```python
from build123d import *

# Parameters (mm, degrees)
F0_W      = 160
F0_H      = 35
F1_DEPTH  = 5
F3_D      = 4.5
F5_R      = 9
F6_DEPTH  = 20
F8_DEPTH  = 25
F9_W      = 15
F9_H      = 2
F10_DEPTH = 20
F12_D     = 4.5
F12_DEPTH = 12
F12_TIP   = 1.3519363928


with BuildPart() as f1:
    # F0 (on Top) → F1 (new body)
    with BuildSketch(Plane.XY):
        with Locations((80, 17.5)):
            Rectangle(F0_W, F0_H)
    extrude(amount=F1_DEPTH)

    # F3 (through all)
    with Locations(Plane(origin=(0, 0, 0), x_dir=(1, 0, 0), z_dir=(0, 0, -1))):
        with Locations((20, -9.5), (60, -9.5), (60, -25.5), (20, -25.5)):
            Hole(F3_D / 2)

    # F5 (on offset) → F6 (join)
    with BuildSketch(Plane.YZ.offset(120)):
        with BuildLine():
            Line((5, 23), (5, 5))
            Line((5, 5), (30, 5))
            Line((30, 5), (30, 23))
            ThreePointArc((30, 23), (17.5, 35.5), (5, 23))
        make_face()
        with Locations((17.5, 23)):
            Circle(F5_R, mode=Mode.SUBTRACT)
    extrude(amount=F6_DEPTH)

    # F7 (on face) → F8 (cut)
    with BuildSketch(Plane.YZ.offset(140)):
        with BuildLine():
            Line((29.9599357944, 24), (26.44427191, 24))
            ThreePointArc((26.44427191, 24), (26.4860571774, 23.5007758031), (26.5, 23))
            ThreePointArc((26.5, 23), (26.4860571774, 22.4992241969), (26.44427191, 22))
            Line((26.44427191, 22), (30, 22))
            Line((30, 22), (30, 23))
            ThreePointArc((30, 23), (29.9899799325, 23.5004011242), (29.9599357944, 24))
        make_face()
    extrude(amount=-F8_DEPTH, mode=Mode.SUBTRACT)

    # F9 (on offset) → F10 (join)
    with BuildSketch(Plane.YZ.offset(120)):
        with Locations((36, 21)):
            Rectangle(F9_W, F9_H)
        with Locations((36, 25)):
            Rectangle(F9_W, F9_H)
    extrude(amount=F10_DEPTH)

    # F12
    with Locations(Plane.XY.offset(26)):
        with Locations((130, 36)):
            Hole(F12_D / 2, depth=F12_DEPTH)
            with Locations((0, 0, -(F12_DEPTH + F12_TIP / 2))):  # 118° drill point
                Cone(0, F12_D / 2, F12_TIP, mode=Mode.SUBTRACT)


solid = f1.part
```
Can you work these out from the model? Positions are in its coordinate system, mm. A direction names the side the tool comes from. Round coordinates to 2 decimals unless told otherwise and drop trailing zeros. Loops run counter-clockwise (first coordinate to the right, second up) from the corner with the lowest first, then second, coordinate; pieces in that order, holes last. Notation, with made-up numbers: (60, 34.5) -> (97, 34.5) arc R20 cw to (97, 64.5) -> close; hole circle Ø1 at (31.5, 10.25). An arc over 180 degrees is marked (long way). Answer in a Markdown table with one row per item.
Item 1: Will these pins go through, and if not, where does the flat tip stop? P1, Ø14.5, axis at x = 132.5, z = 13.5, coming from the -Y side; P2, Ø4, axis at x = 60, y = 25.5, coming from the +Z side; P3, Ø3, axis at x = 135, y = 9, coming from the +Z side; P4, Ø4, axis at x = 126.5, y = 35.5, coming from the +Z side.
Answer block:
| item | result |
|---|---|
| P1 | y = 5 |
| P2 | through |
| P3 | z = 33.36 |
| P4 | z = 26 |
Item 2: On a 3-axis mill with a long thin cutter (end or side, diameter ignored), from which of +Z, -Z, +X, -X, +Y, -Y can I reach the whole of each face in a straight line? I mean faces 5 (the flat face through (127.6, 36.7, 20)), 6 (the flat face through (130, 5, 14)), 7 (the flat face through (127.6, 36.5, 26)), 8 (the cylindrical face through (127.854, 36.676, 20.986)), 9 (the flat face through (79, 0, 2)). Say none if no direction works.
Answer block:
| item | result |
|---|---|
| face 5 | +X, -X, +Y |
| face 6 | +Z, +X, -X, -Y |
| face 7 | +Z, +X, -X, +Y |
| face 8 | +Z |
| face 9 | +Z, -Z, +X, -X, -Y |
Item 3: Suppose I cut it at B-B, the plane y = 40. List the corners of the cut face in (x, z) for me.
Answer block:
| item | result |
|---|---|
| outline | (120, 20) -> (140, 20) -> (140, 22) -> (120, 22) -> close; (120, 24) -> (140, 24) -> (140, 26) -> (120, 26) -> close |
Item 4: Suppose I cut it at C-C, the plane z = 17. List the corners of the cut face in (x, y) for me.
Answer block:
| item | result |
|---|---|
| outline | (120, 5) -> (140, 5) -> (140, 10.79) -> (120, 10.79) -> close; (120, 24.21) -> (140, 24.21) -> (140, 30) -> (120, 30) -> close |
Item 5: Suppose I cut it at A-A, the plane x = 130. List the corners of the cut face in (y, z) for me.
Answer block:
| item | result |
|---|---|
| outline | (0, 0) -> (35, 0) -> (35, 5) -> (30, 5) -> (30, 20) -> (33.75, 20) -> (33.75, 22) -> (26.44, 22) arc R9 cw (long way) to (26.44, 24) -> (33.75, 24) -> (33.75, 26) -> (29.63, 26) arc R12.5 ccw to (5, 23) -> (5, 5) -> (0, 5) -> close; (38.25, 20) -> (43.5, 20) -> (43.5, 22) -> (38.25, 22) -> close; (38.25, 24) -> (43.5, 24) -> (43.5, 26) -> (38.25, 26) -> close |
Item 6: Suppose I cut it at D-D, the plane x = 20. List the corners of the cut face in (y, z) for me, plus the area to 3 significant figures.
Answer block:
| item | result |
|---|---|
| outline | (0, 0) -> (7.25, 0) -> (7.25, 5) -> (0, 5) -> close; (11.75, 0) -> (23.25, 0) -> (23.25, 5) -> (11.75, 5) -> close; (27.75, 0) -> (35, 0) -> (35, 5) -> (27.75, 5) -> close |
| area | 130 mm² |
Item 7: If I drill on probe 1 along Y at (x, z) = (60, 2.6); probe 2 along Y at (x, z) = (130, 24.8); probe 3 along Y at (x, z) = (27.5, 4), over which ranges is the centre line in solid material (lowest first)?
Answer block:
| item | result |
|---|---|
| probe 1 | 0 to 7.25, 11.75 to 23.25, 27.75 to 35 |
| probe 2 | 5.13 to 8.68, 26.32 to 33.75, 38.25 to 43.5 |
| probe 3 | 0 to 35 |
Item 8: We'd pull the mould along X, two halves only. Please class faces 1 (the cylindrical face through (61.786, 26.869, 2.535)), 2 (the cylindrical face through (127.854, 36.676, 24.986)), 3 (the flat face through (79, 18, 0)), 4 (the flat face through (120, 20, 14)): released by +X, released by -X, zero draft, split by the parting line, or undercut.
Answer block:
| item | result |
|---|---|
| face 1 | undercut |
| face 2 | undercut |
| face 3 | zero draft |
| face 4 | released by -X |
